The model under review builds one solid part; all positions refer to its coordinate system, in mm. A direction names the side the tool comes from. Round coordinates to 2 decimals unless told otherwise and drop trailing zeros. Loops run counter-clockwise (first coordinate to the right, second up) from the corner with the lowest first, then second, coordinate; pieces in that order, holes last. Notation, with made-up numbers: M 55.5,79.5 L 84.5,79.5 A25 cw 84.5,108.5 Z; hole C 18.25,37 d6. An arc over 180 degrees is marked long. Return JSON: item names as keys, results as strings. Group by question number.
Q1. For faces 1 (the face through (-47, 48.985, 5)), 2 (the face through (-44, -50, 0)), 3 (the face through (-72, 2.5, 5)), list the 3-axis set-ups (+Z, -Z, +X, -X, +Y, -Y) from which the entire face can be reached by the end or side of a thin tool; tool diameter is ignored.
Q2. Consider section C-C (z = 3). State the section outline as (x, y) points, and give its area (3 significant figures).
Q3. Draft analysis for pull direction X (two halves, no side actions). For faces 4 (the face through (-64.98, 29.06, 4.93)), 5 (the face through (-72, -2.5, 5)), state which applies: pulls with the +X half, pulls with the -X half, needs draft (parallel to the pull), parting line crosses it, or undercut.
Q4. Consider section B-B (y = 0). State the section outline as (x, z) points.
Q5. Clearance check with flat-ended pins moving along their axes: pin 1 Ø3 at (y, z) = (-2.5, 7) entering from +X; pin 2 Ø2 at (x, z) = (-41, 4) entering from -Y; pin 3 Ø4 at (x, z) = (25, 6) entering from +Y. State where each tip first meets the part, or that it passes through.
Q6. To check wall thickness, follow line 1 along X through (y, z) = (1.5, 6.5); line 2 along Y through (x, z) = (48, 5); line 3 along Y through (x, z) = (7.5, 1.75). State the ranges of each line that lie inside material, in increasing order.
Q7. Consider section A-A (x = 0). State the section outline as (y, z) points.
from build123d import *

# Parameters (mm, degrees)
BOSS_EXTRUDE1_DEPTH = 10
BOSS_EXTRUDE2_DEPTH = 10


with BuildPart() as part:
    # Sketch1 → Boss-Extrude1 (new body)
    with BuildSketch(Plane(origin=(0, 0, 0), x_dir=(0, 1, 0), z_dir=(0, 0, 1))):
        with BuildLine():
            Line((-2.500306968, 75.158422449), (-2.500306968, 71.139205273))
            Line((-2.500306968, 71.139205273), (-2.500306968, 69.139205273))
            Line((-2.500306968, 69.139205273), (2.500252848, 69.139205273))
            Line((2.500252848, 69.139205273), (2.500252848, 71.139196387))
            Line((2.500252848, 71.139196387), (2.500252848, 75.15842425))
            ThreePointArc((2.500252848, 75.15842425), (2.7075e-05, -75.2), (-2.500306968, 75.158422449))
        make_face()
        with BuildLine():
            Line((-6.501119998, 70.885625945), (-6.501119998, 65.138162172))
            Line((-6.501119998, 65.138162172), (6.502991614, 65.138162172))
            Line((6.502991614, 65.138162172), (6.502991614, 70.885454269))
            ThreePointArc((6.502991614, 70.885454269), (-0.000939736, -71.18311967), (-6.501119998, 70.885625945))
        make_face(mode=Mode.SUBTRACT)
    extrude(amount=BOSS_EXTRUDE1_DEPTH)

    # Sketch3 → Boss-Extrude2 (add)
    with BuildSketch(Plane.XY.offset(10)):
        Polygon((42.999947541, -53.014633283), (42.999947541, -49.014633283), (55.729863476, -49.014633283), (38.999947541, -62.774922679), (38.999947541, -53.014633283), align=None)
        Polygon((42.999947541, 52.985366717), (42.999947541, 48.985366717), (54.948623561, 48.985366717), (38.999947541, 61.804425072), (38.999947541, 52.985366717), align=None)
        Polygon((-43.000052459, 52.985366717), (-39.000052459, 52.985366717), (-39.000052459, 61.804425072), (-54.585609019, 48.985366717), (-43.000052459, 48.985366717), align=None)
        Polygon((-43.000052459, -53.014633283), (-39.000052459, -53.014633283), (-39.000052459, -62.774922679), (-54.585609019, -49.014633283), (-43.000052459, -49.014633283), align=None)
    extrude(amount=-BOSS_EXTRUDE2_DEPTH)


solid = part.part
Values:
{
 "1": {"face 1": "+Z, -Z", "face 2": "-Z, +X, -X, +Y, -Y", "face 3": "+Z, -Z, -X"},
 "2": {"outline": "M -75.16,-2.5 A75.2 ccw long -75.16,2.5 L -69.14,2.5 L -69.14,-2.5 Z; hole M -70.89,-6.5 A71.18 ccw -51.62,-49.01 L -43,-49.01 L -43,-53.01 L -39,-53.01 L -39,-59.55 A71.18 ccw 39,-59.55 L 39,-53.01 L 43,-53.01 L 43,-49.01 L 51.62,-49.01 A71.18 ccw 51.65,48.99 L 43,48.99 L 43,52.99 L 39,52.99 L 39,59.55 A71.18 ccw -39,59.55 L -39,52.99 L -43,52.99 L -43,48.99 L -51.65,48.99 A71.18 ccw -70.89,6.5 L -65.14,6.5 L -65.14,-6.5 Z", "area": "2,120 mm2"},
 "3": {"face 4": "undercut", "face 5": "needs draft"},
 "4": {"outline": "M -69.14,0 L -65.14,0 L -65.14,10 L -69.14,10 Z; M 71.18,0 L 75.2,0 L 75.2,10 L 71.18,10 Z"},
 "5": {"pin 1": "stops at x = 75.19", "pin 2": "stops at y = -63.68", "pin 3": "stops at y = 71.6"},
 "6": {"line 1": "x = -69.14 to -65.14, 71.17 to 75.19", "line 2": "y = -57.89 to -49.01, 48.99 to 57.89", "line 3": "y = -74.83 to -70.79, 70.79 to 74.83"},
 "7": {"outline": "M -75.2,0 L -71.18,0 L -71.18,10 L -75.2,10 Z; M 71.18,0 L 75.2,0 L 75.2,10 L 71.18,10 Z"}
}
